```python
from build123d import *

# Parameters (mm, degrees)
ESQUISSE1_R             = 35
ESQUISSE1_R_2           = 11.1
ESQUISSE1_R_3           = 1.65
BOSS_EXTRU_1_DEPTH      = 14
BOSS_EXTRU_5_START      = 20
ESQUISSE2_R             = 35
ESQUISSE2_R_2           = 29.905514519
BOSS_EXTRU_5_DEPTH      = 20
BOSS_EXTRU_6_START      = 10
ESQUISSE5_R             = 37.5
ESQUISSE5_R_2           = 29.905514519
BOSS_EXTRU_6_DEPTH      = 10
CONG_1_R                = 10
BOSS_EXTRU_7_START      = 5
ESQUISSE6_R             = 29.905514519
BOSS_EXTRU_7_DEPTH      = 5
ESQUISSE7_R             = 30
ENL_V_MAT_EXTRU_1_DEPTH = 3


with BuildPart() as part:
    # Esquisse1 → Boss.-Extru.1 (new body)
    with BuildSketch(Plane.XY):
        Circle(ESQUISSE1_R)
        Circle(ESQUISSE1_R_2, mode=Mode.SUBTRACT)
        with Locations((-15.5, 15.5)):
            Circle(ESQUISSE1_R_3, mode=Mode.SUBTRACT)
        with Locations((15.5, 15.5)):
            Circle(ESQUISSE1_R_3, mode=Mode.SUBTRACT)
        with Locations((15.5, -15.5)):
            Circle(ESQUISSE1_R_3, mode=Mode.SUBTRACT)
        with Locations((-15.5, -15.5)):
            Circle(ESQUISSE1_R_3, mode=Mode.SUBTRACT)
    extrude(amount=BOSS_EXTRU_1_DEPTH)

    # Esquisse2 → Boss.-Extru.5 (add)
    with BuildSketch(Plane(origin=(0, 0, 0), x_dir=(-1, 0, 0), z_dir=(0, 0, -1)).offset(BOSS_EXTRU_5_START)):
        Circle(ESQUISSE2_R)
        Circle(ESQUISSE2_R_2, mode=Mode.SUBTRACT)
    extrude(amount=-BOSS_EXTRU_5_DEPTH)

    # Esquisse5 → Boss.-Extru.6 (add)
    with BuildSketch(Plane(origin=(0, 0, -20), x_dir=(-1, 0, 0), z_dir=(0, 0, -1)).offset(BOSS_EXTRU_6_START)):
        Circle(ESQUISSE5_R)
        Circle(ESQUISSE5_R_2, mode=Mode.SUBTRACT)
    extrude(amount=-BOSS_EXTRU_6_DEPTH)

    # Congé1
    # the kernel refuses this fillet: 10 mm, written as the material it adds along each edge
    with BuildSketch(Plane(origin=(0, 0, -20), x_dir=(-1, 0, 0), z_dir=(0, -1, 0))) as cong_1_piece_1:
        with BuildLine():
            CenterArc((45, -6.614378278), CONG_1_R, 138.590377891, 41.409622109)
            Line((37.5, 0), (37.35, 0.132287566))
            ThreePointArc((37.35, 0.132287566), (36.25, 0.2), (35, 0.2))
            Line((35, 0.2), (34.8, 0))
            Line((34.8, 0), (34.8, -6.614378278))
            Line((34.8, -6.614378278), (35, -6.614378278))
        make_face()
    revolve(axis=Axis((0, 0, -20), (0, 0, -1)))

    # Esquisse6 → Boss.-Extru.7 (add)
    with BuildSketch(Plane(origin=(0, 0, -30), x_dir=(-1, 0, 0), z_dir=(0, 0, -1)).offset(BOSS_EXTRU_7_START)):
        with BuildLine():
            Line((-12.900778772, 37.862513217), (-80, 15))
            Line((-80, 15), (-80, -15))
            Line((-80, -15), (-12.900778772, -37.862513217))
            ThreePointArc((-12.900778772, -37.862513217), (40, 0), (-12.900778772, 37.862513217))
        make_face()
        Circle(ESQUISSE6_R, mode=Mode.SUBTRACT)
    extrude(amount=-BOSS_EXTRU_7_DEPTH)

    # Esquisse7 → Enlèv. mat.-Extru.1 (cut)
    with BuildSketch(Plane.XY.offset(14)):
        Circle(ESQUISSE7_R)
    extrude(amount=-ENL_V_MAT_EXTRU_1_DEPTH, mode=Mode.SUBTRACT)


solid = part.part
```
Read the model definition and answer for the solid it produces. Units are mm, in the model's axes. A direction names the side the tool comes from. Round coordinates to 2 decimals unless told otherwise and drop trailing zeros. Write each loop counter-clockwise with the first axis right and the second up, starting at its lowest first coordinate (ties: lowest second). Pieces come first, ordered by that corner, then holes. Notation, with made-up numbers: (-38.5, -11) -> (-4.5, -11) arc R17 ccw to (-4.5, 14) -> close; hole circle Ø5 at (-19, -28). An arc over 180 degrees is marked (long way). Answer in a Markdown table with one row per item. Add a question column.
1) Find section D-D, the plane z = -11. Determine the outline of the cut face in (x, y), and give its area (3 significant figures).
2) Find section A-A, the plane y = 0. Determine the outline of the cut face in (x, z), and give its area (3 significant figures).
3) Given P1, Ø24, axis at x = -2.5, y = -9.5, coming from the +Z side; P2, Ø2, axis at y = -12.5, z = -11, coming from the -X side; P3, Ø2, axis at x = 15.5, y = 15.5, coming from the +Z side; P4, Ø2, axis at y = -4.5, z = -19.5, coming from the +X side, each flat-ended and moving along its own axis, determine where each tip first touches the part or whether it passes through.
4) Find section B-B, the plane x = 0. Determine the outline of the cut face in (y, z).
5) Determine the mould class of faces 4 (the face through (43, -3, -30)), 5 (the face through (4.88, 37.18, -25.07)), 6 (the face through (5.97, 9.36, 5.42)), 7 (the face through (17.074, -15.004, 5.423)) for opening direction X: pulls with the +X half, pulls with the -X half, needs draft (parallel to the pull), parting line crosses it, or undercut.
6) Find section C-C, the plane z = 8.5. Determine the outline of the cut face in (x, y), and give its area (3 significant figures).
7) Consider line 1 (Y direction, x = 0, z = -21.5); line 2 (Y direction, x = -15.5, z = 7). Determine where each line is inside the solid, lowest interval first.
8) Which of the six approach directions +Z, -Z, +X, -X, +Y, -Y give full straight-line access (tool end or side, diameter ignored) to faces 1 (the face through (13, 0, 11)), 2 (the face through (29.877, 1.315, -17.745)), 3 (the face through (80, 0, -33))?
Findings below:
| question | item | result |
|---|---|---|
| 1 | outline | circle Ø70 at (0, 0); hole circle Ø59.81 at (0, 0) |
| 1 | area | 1,040 mm² |
| 2 | outline | (-40, -35) -> (-29.91, -35) -> (-29.91, 0) -> (-11.1, 0) -> (-11.1, 11) -> (-30, 11) -> (-30, 14) -> (-35, 14) -> (-35, -13.39) arc R10 cw to (-37.5, -20) -> (-37.5, -30) -> (-40, -30) -> close; (11.1, 0) -> (29.91, 0) -> (29.91, -35) -> (80, -35) -> (80, -30) -> (37.5, -30) -> (37.5, -20) arc R10 cw to (35, -13.39) -> (35, 14) -> (30, 14) -> (30, 11) -> (11.1, 11) -> close |
| 2 | area | 1,220 mm² |
| 3 | P1 | z = 11 |
| 3 | P2 | x = -33.06 |
| 3 | P3 | through |
| 3 | P4 | x = 37.32 |
| 4 | outline | (-40, -35) -> (-29.91, -35) -> (-29.91, 0) -> (-11.1, 0) -> (-11.1, 11) -> (-30, 11) -> (-30, 14) -> (-35, 14) -> (-35, -13.39) arc R10 cw to (-37.5, -20) -> (-37.5, -30) -> (-40, -30) -> close; (11.1, 0) -> (29.91, 0) -> (29.91, -35) -> (40, -35) -> (40, -30) -> (37.5, -30) -> (37.5, -20) arc R10 cw to (35, -13.39) -> (35, 14) -> (30, 14) -> (30, 11) -> (11.1, 11) -> close |
| 5 | face 4 | needs draft |
| 5 | face 5 | parting line crosses it |
| 5 | face 6 | undercut |
| 5 | face 7 | undercut |
| 6 | outline | circle Ø70 at (0, 0); hole circle Ø3.3 at (-15.5, -15.5); hole circle Ø3.3 at (-15.5, 15.5); hole circle Ø22.2 at (0, 0); hole circle Ø3.3 at (15.5, -15.5); hole circle Ø3.3 at (15.5, 15.5) |
| 6 | area | 3,430 mm² |
| 7 | line 1 | -37.5 to -29.91, 29.91 to 37.5 |
| 7 | line 2 | -31.38 to -17.15, -13.85 to 13.85, 17.15 to 31.38 |
| 8 | face 1 | +Z |
| 8 | face 2 | -Z |
| 8 | face 3 | +Z, -Z, +X, +Y, -Y |
